Design review of the part built by this model. Coordinates are the model's own, in mm. Face numbers are marked on the shaded views. A direction names the side the tool comes from. Give positions to 0.01 mm unless a question says otherwise; leave off trailing zeros. Loops run counter-clockwise (first coordinate to the right, second up) from the corner with the lowest first, then second, coordinate; pieces in that order, holes last. Notation, with made-up numbers: (11.25, 35.5) - (60.25, 35.5) arc R23 cw to (60.25, 49.5) - close; hole circle Ø7 at (43.5, -19.75). An arc over 180 degrees is marked (long way). Write each question's results on one line, items separated by ' | '.
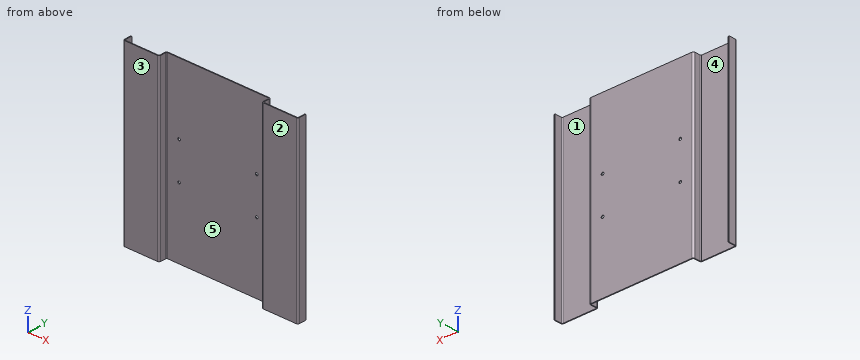
Autodesk Inventor part; units mm, degrees
ref_plane "YZ Plane" through (0, 0, 0) normal (1, 0, 0) x (0, 1, 0)
ref_plane "XZ Plane" through (0, 0, 0) normal (0, 1, 0) x (-1, 0, 0)
ref_plane "XY Plane" through (0, 0, 0) normal (0, 0, 1) x (1, 0, 0)
sketch "Sketch1" plane through (0, 0, 0) normal (0, 1, 0) x (-1, 0, 0)
  line L0 (-59, -98) -> (59, -98)
  line L1 (59, -98) -> (59, 98)
  line L2 (59, 98) -> (-59, 98)
  line L3 (-59, 98) -> (-59, -98)
  line L4 (-59, -98) -> (59, 98) construction
  line L5 (59, -98) -> (-59, 98) construction
  point P0 (0, 0)
  dimension "d0" = 118
  dimension "d1" = 196
extrude "Plate1" add sketch "Sketch1" along normal blind 0.9119
sketch "Sketch2" plane through (58.0881, 0.9119, 98) normal (1, 0, 0) x (0, 1, 0)
  line L0 (0, -196) -> (0, 0)
  line L1 (0, 0) -> (-10, 0)
  line L2 (-10, 0) -> (-10, -196)
  line L3 (-10, -196) -> (0, -196)
edge flange "Flange1" height 10 angle 90 thickness 0.9119 bend radius 0.9119 thickness toward (1, 0, 0) relief tear relief width 0.9119 relief depth 0.4559 corner gap 0.9119 corner form 0 edges at (59, 0, 0) (-59, 0, 0) wall of the first edge with corners at (58.0881, 0.9119, -98) (58.0881, 0.9119, 98) (58.0881, -9.0881, 98) (58.0881, -9.0881, -98)
bend "Bend1"
corner "Corner1"
sketch "Sketch3" plane through (58.0881, -8.1763, -98) normal (0, -1, 0) x (1, 0, 0)
  line L0 (0, 196) -> (0, 0)
  line L1 (0, 0) -> (40, 0)
  line L2 (40, 0) -> (40, 196)
  line L3 (40, 196) -> (0, 196)
edge flange "Flange2" height 40 angle 90 thickness 0.9119 bend radius 0.9119 thickness toward (0, -1, 0) relief tear relief width 0.9119 relief depth 0.4559 corner gap 0.9119 corner form 0 edges at (59, -9.0881, 0) (-59, -9.0881, 0) wall of the first edge with corners at (58.0881, -8.1763, 98) (58.0881, -8.1763, -98) (98.0881, -8.1763, -98) (98.0881, -8.1763, 98)
bend "Bend2"
corner "Corner2"
sketch "Sketch4" plane through (98.0881, -8.1763, -98) normal (1, 0, 0) x (0, 1, 0)
  line L0 (0, 196) -> (0, 0)
  line L1 (0, 0) -> (9.0881, 0)
  line L2 (9.0881, 0) -> (9.0881, 196)
  line L3 (9.0881, 196) -> (0, 196)
edge flange "Flange3" height 10 angle 90 thickness 0.9119 bend radius 0.9119 thickness toward (1, 0, 0) relief tear relief width 0.9119 relief depth 0.4559 corner gap 0.9119 corner form 0 edges at (98.0881, -8.1763, 0) (-98.0881, -8.1763, 0) wall of the first edge with corners at (98.0881, -8.1763, 98) (98.0881, -8.1763, -98) (98.0881, 0.9119, -98) (98.0881, 0.9119, 98)
bend "Bend3"
corner "Corner3"
sketch "Sketch5" plane through (0, 0.9119, 0) normal (0, 1, 0) x (1, 0, 0)
  line L0 (0, 0) -> (-59, 0)
  line L1 (-59, 0) -> (-59, 98)
  line L2 (-59, 98) -> (0, 98)
  line L3 (0, 98) -> (0, 0)
  line L4 (140, -28) -> (-140, -28)
  line L5 (-140, -28) -> (-140, 28)
  line L6 (-140, 28) -> (140, 28)
  line L7 (140, 28) -> (140, -28)
  line L8 (140, -28) -> (-140, 28) construction
  line L9 (-140, -28) -> (140, 28) construction
  circle A0 centre (-44, 20.5) radius 1.5
  circle A1 centre (44, 20.5) radius 1.5
  circle A2 centre (-44, -20.5) radius 1.5
  circle A3 centre (44, -20.5) radius 1.5
  dimension "d34" = 280
  dimension "d35" = 56
  dimension "d36" = 3
  dimension "d38" = 44
  dimension "d41" = 20.5
extrude "Cut1" cut sketch "Sketch5" against normal blind 0.9119 contours A0 | A1 | A2 | A3
fillet "Corner Round1" radius 1 4 edges at (-98.5441, 0.9119, 98) (-98.5441, 0.9119, -98) (98.5441, 0.9119, -98) (98.5441, 0.9119, 98)
equation "\"d0\" = foot_x - 2 * frame_border"
equation "\"d1\" = foot_y"
equation "\"d34\" = frame_front_x"
equation "\"d35\" = frame_front_y"
equation "\"d36\" = m3_diameter"
equation "\"d38\" = laser_offset_x - frame_front_fold"
equation "\"d41\" = 0.5 * frame_front_y - 0.5 * frame_front_fold"
equation "\"d39\" = Thickness"
equation "\"d33\" = corner_small_r"
equation "\"Thickness\" = foot_t"
equation "\"d3\" = BendReliefWidth"
equation "\"d4\" = BendReliefDepth"
equation "\"d5\" = MinimumRemnant"
equation "\"d6\" = BendRadius"
equation "\"d7\" = foot_z"
equation "\"d9\" = BendRadius"
equation "\"d10\" = CornerReliefSize"
equation "\"d11\" = GapSize"
equation "\"d12\" = JacobiRadiusSize"
equation "\"d13\" = BendReliefWidth"
equation "\"d14\" = BendReliefDepth"
equation "\"d15\" = MinimumRemnant"
equation "\"d16\" = BendRadius"
equation "\"d17\" = frame_border"
equation "\"d19\" = BendRadius"
equation "\"d20\" = CornerReliefSize"
equation "\"d21\" = GapSize"
equation "\"d22\" = JacobiRadiusSize"
equation "\"d23\" = BendReliefWidth"
equation "\"d24\" = BendReliefDepth"
equation "\"d25\" = MinimumRemnant"
equation "\"d26\" = BendRadius"
equation "\"d27\" = foot_z"
equation "\"d29\" = BendRadius"
equation "\"d30\" = CornerReliefSize"
equation "\"d31\" = GapSize"
equation "\"d32\" = JacobiRadiusSize"
equation "\"BendRadius\" = Thickness"
equation "\"BendReliefWidth\" = Thickness"
equation "\"BendReliefDepth\" = 0.5 * Thickness"
equation "\"CornerReliefSize\" = 4 * Thickness"
equation "\"MinimumRemnant\" = 2 * Thickness"
equation "\"TransitionRadius\" = BendRadius"
equation "\"JacobiRadiusSize\" = BendRadius"
equation "\"GapSize\" = Thickness"
equation "\"laserresin\" = 5"
equation "\"st1_thickness\" = 0.91186"
equation "\"st2_thickness\" = 1.5875"
equation "\"al1_thickness\" = 0.79375"
equation "\"al2_thickness\" = 1.5875"
equation "\"bend_factor\" = 2.26205"
equation "\"st1_bend\" = 2.06267"
equation "\"st2_bend\" = 3.591"
equation "\"st3_bend\" = 113.10236"
equation "\"al1_bend\" = 1.7955"
equation "\"al2_bend\" = 3.591"
equation "\"al3_bend\" = 113.10236"
equation "\"acrylic1_thickness\" = 5.88"
equation "\"acrylic2_thickness\" = 3.15"
equation "\"acrylic3_thickness\" = 3.15"
equation "\"corner_small_r\" = 1"
equation "\"corner_big_r\" = 5"
equation "\"linear_bearing_spacing\" = 208"
equation "\"galvo_y_out_offset\" = 27"
equation "\"galvo_y_in_offset\" = 17.5"
equation "\"laser_diameter\" = 13"
equation "\"nema17_x\" = 43"
equation "\"nema17_shaft\" = 24"
equation "\"lmk8uu_x\" = 25"
equation "\"lmk8uu_shaft\" = 15"
equation "\"lmk8uu_z\" = 24"
equation "\"shf8_y\" = 43"
equation "\"acme_nut_d\" = 19.1"
equation "\"acme_nut_upper_d\" = 12.7"
equation "\"handle_spacing\" = 50.8"
equation "\"handle_d\" = 4.7625"
equation "\"handle_hole_d\" = 2.845"
equation "\"handle_projection\" = 20.6375"
equation "\"switch_spacing\" = 19"
equation "\"laser_body_diameter\" = 12"
equation "\"m3_diameter\" = 3"
equation "\"m3_head\" = 6"
equation "\"m4_diameter\" = 4"
equation "\"m5_diameter\" = 5"
equation "\"m5_head\" = 10.3"
equation "\"rivet1_diameter\" = 3.26"
equation "\"rivet2_diameter\" = 3.26"
equation "\"brass_insert_drill\" = 4"
equation "\"m5_brass_insert_drill\" = 6.7"
equation "\"m3_press_nut_drill\" = 4.24"
equation "\"m5_press_nut_drill\" = 6.35"
equation "\"platform_t\" = 1.5875"
equation "\"platform_z\" = 65"
equation "\"platform_fold_x\" = 15"
equation "\"platform_crane_gap\" = 0.1"
equation "\"platform_gap\" = 0.1"
equation "\"platform_upper_y\" = 46.625"
equation "\"crane_t\" = 1.5875"
equation "\"crane_x\" = 233"
equation "\"crane_gap\" = 0.1"
equation "\"tray_t\" = 5.88"
equation "\"tray_to_platform_oversize\" = 0"
equation "\"reservoir_t\" = 0.91186"
equation "\"reservoir_z\" = 35"
equation "\"reservoir_flap_y\" = 20.91186"
equation "\"frame_front_t\" = 0.91186"
equation "\"frame_front_x\" = 280"
equation "\"frame_front_y\" = 56"
equation "\"frame_front_fold\" = 15"
equation "\"frame_gap\" = 0.1"
equation "\"frame_back_t\" = 0.91186"
equation "\"frame_back_x\" = 277.97628"
equation "\"frame_back_y\" = 53.97628"
equation "\"frame_back_z\" = 497.97628"
equation "\"drawer_t\" = 0.91186"
equation "\"drawer_gap\" = 0.1"
equation "\"drawer_reservoir_overlap_x\" = 24.08814"
equation "\"drawer_x\" = 202.02372"
equation "\"drawer_y\" = 73"
equation "\"drawer_seal_y\" = 101"
equation "\"drawer_window_gap\" = 6"
equation "\"foot_t\" = 0.91186"
equation "\"foot_x\" = 198"
equation "\"foot_y\" = 196"
equation "\"laser_holder_t\" = 0.91186"
equation "\"laser_holder_z\" = 75"
equation "\"laser_offset_x\" = 59"
equation "\"laser_offset_y\" = 8.5"
equation "\"subframe_t\" = 0.79375"
equation "\"subframe_x\" = 66"
equation "\"subframe_y\" = 55"
equation "\"d2\" = BendRadius"
equation "\"shield_y\" = 71"
equation "\"shield_x\" = 200.2"
equation "\"shield_z\" = 259.9"
equation "\"shield_t\" = 3.15"
equation "\"magnet_t\" = 1.6"
equation "\"magnet_w\" = 12.8"
equation "\"sae_4_40_diameter\" = 2.845"
properties part number "foot" material "Steel, Mild"
(1) Take a section at A-A on y = -3. Give the boundary of the cut face in (x, z).
Answers below:
outline: (-99, -98) - (-98.09, -98) - (-98.09, 98) - (-99, 98) - close; (-59, -98) - (-58.09, -98) - (-58.09, 98) - (-59, 98) - close; (58.09, -98) - (59, -98) - (59, 98) - (58.09, 98) - close; (98.09, -98) - (99, -98) - (99, 98) - (98.09, 98) - close
(2) Tool access review of the marked faces 3, 4 and 5: name each direction out of +Z, -Z, +X, -X, +Y, -Y from which nothing blocks a thin tool from reaching the whole face with its end or side.
Answers below:
face 3: +Z, -Z, +X, -X, -Y | face 4: +Z, -Z, +Y | face 5: +Z, -Z, -Y
(3) Take a section at C-C on x = 74.5. Give the boundary of the cut face in (y, z).
Answers below:
outline: (-9.09, -98) - (-8.18, -98) - (-8.18, 98) - (-9.09, 98) - close
(4) Take a section at B-B on z = 49. Give the boundary of the cut face in (x, y), plus the area to 3 significant figures.
Answers below:
outline: (-99, -7.26) arc R1.82 ccw to (-97.18, -9.09) - (-59.91, -9.09) arc R1.82 ccw to (-58.09, -7.26) - (-58.09, -0.91) arc R0.91 cw to (-57.18, 0) - (57.18, 0) arc R0.91 cw to (58.09, -0.91) - (58.09, -7.26) arc R1.82 ccw to (59.91, -9.09) - (97.18, -9.09) arc R1.82 ccw to (99, -7.26) - (99, 0.91) - (98.09, 0.91) - (98.09, -7.26) arc R0.91 cw to (97.18, -8.18) - (59.91, -8.18) arc R0.91 cw to (59, -7.26) - (59, -0.91) arc R1.82 ccw to (57.18, 0.91) - (-57.18, 0.91) arc R1.82 ccw to (-59, -0.91) - (-59, -7.26) arc R0.91 cw to (-59.91, -8.18) - (-97.18, -8.18) arc R0.91 cw to (-98.09, -7.26) - (-98.09, 0.91) - (-99, 0.91) - close | area: 210 mm2
(5) Wall thickness on line 1 along Z through (x, y) = (44, 0.7); line 2 along X through (y, z) = (-2.5, -43.5); line 3 along X through (y, z) = (0.25, 20.5): over which ranges is each line inside the solid? List them lowest first. Write a range as from..to.
Answers below:
line 1: -98..-22, -19..19, 22..98 | line 2: -99..-98.09, -59..-58.09, 58.09..59, 98.09..99 | line 3: -99..-98.09, -58.58..-45.5, -42.5..42.5, 45.5..58.58, 98.09..99
(6) Insertion check: P1, Ø2, axis at x = 0, z = -8, coming from the -Y side; P2, Ø2, axis at y = -7.5, z = 31.5, coming from the -X side. Each pin has a flat end and moves straight along its axis. Give the tip position at first contact, or say it passes through.
Answers below:
P1: y = 0 | P2: x = -99
(7) Draft analysis for pull direction X (two halves, no side actions). For the marked faces 1 and 2, state which applies: pulls with the +X half, pulls with the -X half, needs draft (parallel to the pull), parting line crosses it, or undercut.
Answers below:
face 1: undercut | face 2: needs draft
